For this review, take the finished solid that the model builds, in its own axes (mm). Face numbers are marked on the shaded views. A direction names the side the tool comes from. Coordinates: 2 decimals unless noted, no trailing zeros. Write each loop counter-clockwise with the first axis right and the second up, starting at its lowest first coordinate (ties: lowest second). Pieces come first, ordered by that corner, then holes. Notation, with made-up numbers: (-25.75, 78) -> (-11.75, 78) arc R9 ccw to (-11.75, 87) -> close; hole circle Ø3 at (21, 15). An arc over 180 degrees is marked (long way). Put each result on its own line as item: value. Start each with the question number.
Item 1: Consider section C-C on z = 277. Give the boundary of the cut face in (x, y), and give its area (3 significant figures).
Item 2: Consider section B-B on z = 151. Give the boundary of the cut face in (x, y).
Item 3: To check wall thickness, follow L1, parallel to Z at x = 64, y = 56; L2, parallel to Z at x = -44, y = 104; L3, parallel to X at y = 36, z = 140. State the ranges of each line that lie inside material, in increasing order.
Item 4: For the marked faces 4, 5, 6, 7 and 8, list the 3-axis set-ups (+Z, -Z, +X, -X, +Y, -Y) from which the entire face can be reached by the end or side of a thin tool; tool diameter is ignored.
Item 5: Consider section A-A on x = -105. Give the boundary of the cut face in (y, z).
Item 6: The part is to be moulded in two halves that separate along Z. For the marked faces 1, 2 and 3, say which applies: +Z half, -Z half, draft (parallel to the pull), parting line (faces both ways), or undercut.
Item 7: Consider section D-D on y = 99.5. Give the number of separate pieces and of enclosed holes in the cut face, and give its area (3 significant figures).
Item 8: Insertion check: P1, Ø3, axis at x = -212.5, z = 281, coming from the -Y side; P2, Ø1, axis at y = -58.5, z = 177.5, coming from the +X side; P3, Ø2, axis at x = 11.5, z = 204, coming from the +Y side; P4, Ø25, axis at x = 63, z = 104.5, coming from the +Y side. Each pin has a flat end and moves straight along its axis. Give the tip position at first contact, or say it passes through.
```python
from build123d import *
from OCP.BRepFilletAPI import BRepFilletAPI_MakeChamfer

# Parameters (mm, degrees)
BOSS_EXTRU_1_DEPTH      = 320
ENL_V_MAT_EXTRU_1_DEPTH = 30
ENL_V_START             = -295
ENL_V_MAT_EXTRU_2_DEPTH = 25
ESQUISSE5_R             = 26
BOSS_EXTRU_2_DEPTH      = 20
BOSS_EXTRU_3_START      = -35
ESQUISSE5_3_R           = 50
BOSS_EXTRU_3_DEPTH      = 40
BOSS_EXTRU_4_START      = -300
ESQUISSE5_5_R           = 50
BOSS_EXTRU_4_DEPTH      = 20
BOSS_EXTRU_5_START      = -300
ESQUISSE5_6_R           = 26
BOSS_EXTRU_5_DEPTH      = 20
CHANFREIN1_SIZE         = 5
CHANFREIN1_SIZE_2       = 6.671835022
CHANFREIN2_SIZE         = 5
CHANFREIN2_SIZE2        = 6.671835022
CHANFREIN2_SIZE2_2      = 4.169025226
CHAMFER1_START          = 179.129452599
CHAMFER1_OUTLINE_W      = 53
CHAMFER1_OUTLINE_H      = 22
CHAMFER1_DEPTH          = 6.870547401
CHAMFER3_START          = 179.129452599
CHAMFER3_OUTLINE_W      = 53
CHAMFER3_OUTLINE_H      = 22
CHAMFER3_DEPTH          = 6.870547401


with BuildPart() as part:
    # Esquisse1 → Boss.-Extru.1 (new body)
    with BuildSketch(Plane.XY):
        Polygon((10.109909982, 160.217391304), (45.109909982, 160.217391304), (-12.607137799, -89.782608696), (-47.607137799, -89.782608696), align=None)
    extrude(amount=BOSS_EXTRU_1_DEPTH)

    # Esquisse2 → Enlèv. mat.-Extru.1 (cut)
    with BuildSketch(Plane.XY.offset(320)):
        Polygon((-47.607137799, -89.782608696), (-42.989773977, -69.782608696), (-7.989773977, -69.782608696), (-12.607137799, -89.782608696), align=None)
    extrude(amount=-ENL_V_MAT_EXTRU_1_DEPTH, mode=Mode.SUBTRACT)

    # Esquisse3 → Enlèv. mat.-Extru.2 (cut)
    with BuildSketch(Plane.XY.offset(320).offset(ENL_V_START)):
        Polygon((-47.607137799, -89.782608696), (-42.989773977, -69.782608696), (-7.989773977, -69.782608696), (-12.607137799, -89.782608696), align=None)
    extrude(amount=-ENL_V_MAT_EXTRU_2_DEPTH, mode=Mode.SUBTRACT)

    # Esquisse5 → Boss.-Extru.2 (add)
    with BuildSketch(Plane.XY.offset(320)):
        with BuildLine():
            Line((98.109909982, 160.217391304), (45.109909982, 160.217391304))
            Line((45.109909982, 160.217391304), (2.551706555, -24.122440094))
            add(Edge.make_bspline(
                [(98.109909982, 160.217391304), (195.681111268, 92.37740659), (50.514460477, 17.497979542), (2.551706555, -24.122440094)],
                knots=[0, 0, 0, 0, 1, 1, 1, 1], degree=3))
        make_face()
        with Locations((95.109909982, 110.217391304)):
            Circle(ESQUISSE5_R, mode=Mode.SUBTRACT)
    extrude(amount=-BOSS_EXTRU_2_DEPTH)

    # Esquisse5<3> → Boss.-Extru.3 (add)
    with BuildSketch(Plane.XY.offset(320).offset(BOSS_EXTRU_3_START)):
        with BuildLine():
            Line((-230.213971145, -0.950262244), (-40.985726083, -61.102123595))
            Line((-40.985726083, -61.102123595), (10.109909982, 160.217391304))
            Line((10.109909982, 160.217391304), (-187.731895981, 173.717391304))
            ThreePointArc((-187.731895981, 173.717391304), (-277.611698921, 103.077652588), (-230.213971145, -0.950262244))
        make_face()
        with Locations((-187.731895981, 81.217391304)):
            Circle(ESQUISSE5_3_R, mode=Mode.SUBTRACT)
    extrude(amount=-BOSS_EXTRU_3_DEPTH)

    # Esquisse5<5> → Boss.-Extru.4 (add)
    with BuildSketch(Plane.XY.offset(320).offset(BOSS_EXTRU_4_START)):
        with BuildLine():
            Line((-230.213971145, -0.950262244), (-40.985726083, -61.102123595))
            Line((-40.985726083, -61.102123595), (10.109909982, 160.217391304))
            Line((10.109909982, 160.217391304), (-187.731895981, 173.717391304))
            ThreePointArc((-187.731895981, 173.717391304), (-277.611698921, 103.077652588), (-230.213971145, -0.950262244))
        make_face()
        with Locations((-187.731895981, 81.217391304)):
            Circle(ESQUISSE5_5_R, mode=Mode.SUBTRACT)
    extrude(amount=-BOSS_EXTRU_4_DEPTH)

    # Esquisse5<6> → Boss.-Extru.5 (add)
    with BuildSketch(Plane.XY.offset(320).offset(BOSS_EXTRU_5_START)):
        with BuildLine():
            Line((98.109909982, 160.217391304), (45.109909982, 160.217391304))
            Line((45.109909982, 160.217391304), (2.551706555, -24.122440094))
            add(Edge.make_bspline(
                [(98.109909982, 160.217391304), (195.681111268, 92.37740659), (50.514460477, 17.497979542), (2.551706555, -24.122440094)],
                knots=[0, 0, 0, 0, 1, 1, 1, 1], degree=3))
        make_face()
        with Locations((95.109909982, 110.217391304)):
            Circle(ESQUISSE5_6_R, mode=Mode.SUBTRACT)
    extrude(amount=-BOSS_EXTRU_5_DEPTH)

    # Chanfrein1
    # the kernel refuses this chamfer: 6.671835022, 5 mm, written as the material it takes off along each edge
    with BuildSketch(Plane(origin=(10.109909982, 160.217391304, 20), x_dir=(1, 0, 0), z_dir=(0, 0, 1))) as chanfrein1_piece_1:
        Polygon((CHANFREIN1_SIZE, 0), (-CHANFREIN1_SIZE_2 * 0.224951054343, -CHANFREIN1_SIZE_2 * 0.974370064782), (0, 0), align=None)
    extrude(amount=225, mode=Mode.SUBTRACT)
    with BuildSketch(Plane(origin=(10.109909982, 160.217391304, 285), x_dir=(1, 0, 0), z_dir=(0, 0, 1))) as chanfrein1_piece_2:
        Polygon((CHANFREIN1_SIZE, 0), (-CHANFREIN1_SIZE_2 * 0.224951054343, -CHANFREIN1_SIZE_2 * 0.974370064782), (0, 0), align=None)
    extrude(amount=52.24901503, mode=Mode.SUBTRACT)

    # Chanfrein2: one chamfer whose edges measure the first distance from different faces: ONE call of the kernel's chamfer builder (chamfer() names one face for all edges)
    chanfrein2_edges_1 = [part.edges().sort_by_distance(p)[0] for p in [
        (-12.607137799, -89.782608696, 157.5),
    ]]
    chanfrein2_side_1 = [part.faces().sort_by_distance(p)[0] for p in [
        (-30.107137799, -89.782608696, 157.5),
    ]]
    chanfrein2_edges_2 = [part.edges().sort_by_distance(p)[0] for p in [
        (-47.607137799, -89.782608696, 157.5),
    ]]
    chanfrein2_side_2 = [part.faces().sort_by_distance(p)[0] for p in [
        (-19.722598228, 30.998601722, 155.760522115),
    ]]
    chanfrein2 = BRepFilletAPI_MakeChamfer(part.part.solid().wrapped)
    for e in chanfrein2_edges_1:
        chanfrein2.Add(CHANFREIN2_SIZE, CHANFREIN2_SIZE2, e.wrapped, chanfrein2_side_1[0].wrapped)  # the first distance lies on this face
    for e in chanfrein2_edges_2:
        chanfrein2.Add(CHANFREIN2_SIZE, CHANFREIN2_SIZE2_2, e.wrapped, chanfrein2_side_2[0].wrapped)  # the first distance lies on this face
    add(Compound.cast(chanfrein2.Shape()), mode=Mode.REPLACE)

    # Chamfer1: read off the stored shape, not the designer's step
    # Chamfer1 outline → Chamfer1 (cut)
    with BuildSketch(Plane(origin=(0, 0, 0), x_dir=(0.7071067811868629, -0.707106781186232, 0), z_dir=(0.707106781186232, 0.707106781186863, 0)).offset(CHAMFER1_START)):
        with Locations((-22.5, -310)):
            Rectangle(CHAMFER1_OUTLINE_W, CHAMFER1_OUTLINE_H)
    extrude(amount=CHAMFER1_DEPTH, mode=Mode.SUBTRACT)

    # Chamfer3: read off the stored shape, not the designer's step
    # Chamfer3 outline → Chamfer3 (cut)
    with BuildSketch(Plane(origin=(0, 0, 0), x_dir=(0.7071067811868629, -0.707106781186232, 0), z_dir=(0.707106781186232, 0.707106781186863, 0)).offset(CHAMFER3_START)):
        with Locations((-22.5, -10)):
            Rectangle(CHAMFER3_OUTLINE_W, CHAMFER3_OUTLINE_H)
    extrude(amount=CHAMFER3_DEPTH, mode=Mode.SUBTRACT)


solid = part.part
```
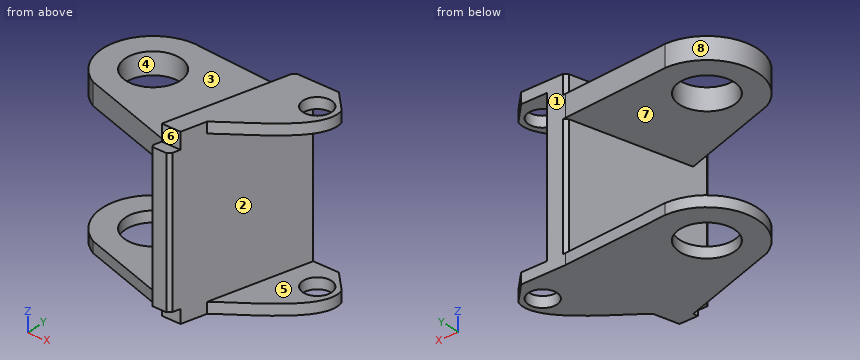
Return value:
1. outline: (-230.21, -0.95) -> (-40.99, -61.1) -> (-46.48, -84.91) -> (-43.44, -89.78) -> (-17.61, -89.78) -> (-11.11, -83.28) -> (45.11, 160.22) -> (10.11, 160.22) -> (-187.73, 173.72) arc R92.5 ccw to start; hole circle Ø100 at (-187.73, 81.22)
1. area: 50,300 mm^2
2. outline: (-46.48, -84.91) -> (-43.44, -89.78) -> (-17.61, -89.78) -> (-11.11, -83.28) -> (45.11, 160.22) -> (15.11, 160.22) -> (8.61, 153.72) -> close
3. L1: 0 to 20, 300 to 320
3. L2: 0 to 20, 245 to 285
3. L3: -18.57 to 16.43
4. face 4: +Z, -Z
4. face 5: +X, -Y
4. face 6: +Z, +X, -X, -Y
4. face 7: -X, +Y
4. face 8: +Z, -Z, -X
5. outline: (-40.75, 0) -> (168.07, 0) -> (168.07, 20) -> (-40.75, 20) -> close; (-40.75, 245) -> (168.07, 245) -> (168.07, 285) -> (-40.75, 285) -> close
6. face 1: draft
6. face 2: undercut
6. face 3: +Z half
7. separate pieces: 5
7. enclosed holes: 0
7. area: 24,100 mm^2
8. P1: y = -7.06
8. P2: x = -5.27
8. P3: y = 157.61
8. P4: through
